from build123d import *

# Parameters (mm, degrees)
F0_R            = 4.05
F1_DEPTH        = 10
F2_R            = 5
F4_D            = 4.1000000042
F4_CSINK_D      = 7.7978
F4_CSINK_ANGLE  = 82
F5_W            = 1
F5_H            = 12
F6_DEPTH        = 0.4
F8_DEPTH        = 25
F10_D           = 3
F10_CBORE_D     = 6.5
F10_CBORE_DEPTH = 3


with BuildPart() as f1:
    # F0 (on Top) → F1 (new body)
    with BuildSketch(Plane.XY):
        Polygon((67.5994434953, -8.2149432153), (-62.4005565047, -8.2149432153), (-62.4005565047, -32.2149432153), (-28.9914757013, -32.2149432153), (-28.9914757013, -20.2149432153), (34.1903626919, -20.2149432153), (34.1903626919, -32.2149432153), (67.5994434953, -32.2149432153), align=None)
        with Locations((-47.4005565047, -20.2149432153)):
            Circle(F0_R, mode=Mode.SUBTRACT)
        with Locations((52.5994434953, -20.2149432153)):
            Circle(F0_R, mode=Mode.SUBTRACT)
    extrude(amount=F1_DEPTH)

    # F2
    f2_edges = [f1.edges().sort_by_distance(p)[0] for p in [
        (34.190363, -32.214943, 5),
        (-28.991476, -32.214943, 5),
    ]]
    fillet(f2_edges, radius=F2_R)

    # F4 (through all)
    with Locations(Plane.XZ.offset(20.2149432153)):
        with Locations((-18.9914757013, 5), (24.1903626919, 5)):
            CounterSinkHole(F4_D / 2, F4_CSINK_D / 2, counter_sink_angle=F4_CSINK_ANGLE)

    # F5 (on face) → F6 (join)
    with BuildSketch(Plane.XY.offset(10)):
        with Locations((2.5994434953, -14.2149432153)):
            Rectangle(F5_W, F5_H)
    extrude(amount=F6_DEPTH)

    # F7 (on face) → F8 (cut)
    with BuildSketch(Plane.XY.offset(10)):
        with BuildLine():
            ThreePointArc((56.6417200816, -19.9649432153), (56.6475121814, -20.0898835784), (56.6494434953, -20.2149432153))
            ThreePointArc((56.6494434953, -20.2149432153), (56.6475121814, -20.3400028521), (56.6417200816, -20.4649432153))
            Line((56.6417200816, -20.4649432153), (67.5994434953, -20.4649432153))
            Line((67.5994434953, -20.4649432153), (67.5994434953, -19.9649432153))
            Line((67.5994434953, -19.9649432153), (56.6417200816, -19.9649432153))
        make_face()
        with BuildLine():
            Line((-51.442833091, -19.9649432153), (-62.4005565047, -19.9649432153))
            Line((-62.4005565047, -19.9649432153), (-62.4005565047, -20.4649432153))
            Line((-62.4005565047, -20.4649432153), (-51.442833091, -20.4649432153))
            ThreePointArc((-51.442833091, -20.4649432153), (-51.4505565047, -20.2149432153), (-51.442833091, -19.9649432153))
        make_face()
        with BuildLine():
            Line((-51.442833091, -20.4649432153), (-51.442833091, -19.9649432153))
            ThreePointArc((-51.442833091, -19.9649432153), (-51.4505565047, -20.2149432153), (-51.442833091, -20.4649432153))
        make_face()
        with BuildLine():
            ThreePointArc((56.6417200816, -20.4649432153), (56.6475121814, -20.3400028521), (56.6494434953, -20.2149432153))
            ThreePointArc((56.6494434953, -20.2149432153), (56.6475121814, -20.0898835784), (56.6417200816, -19.9649432153))
            Line((56.6417200816, -19.9649432153), (56.6417200816, -20.4649432153))
        make_face()
    extrude(amount=-F8_DEPTH, mode=Mode.SUBTRACT)

    # F10 (through all)
    with Locations(Plane.XZ.offset(32.2149432153)):
        with Locations((61.5994434953, 5), (-56.4005565047, 5)):
            CounterBoreHole(F10_D / 2, F10_CBORE_D / 2, F10_CBORE_DEPTH)


solid = f1.part
Geometry: final body of the model. Coordinates: model frame, mm. A direction names the side the tool comes from. Coordinates: 2 decimals unless noted, no trailing zeros. Order: outer loops, then holes, each group sorted by start corner. A loop starts at its lowest first (then second) coordinate and runs counter-clockwise, first axis right, second up.
1) Section B-B (x = -45). Return loops of the section in (y, z), then the cut area to 3 significant figures.
Result sheet:
outline: (-32.21, 0) - (-23.48, 0) - (-23.48, 10) - (-32.21, 10) - close; (-16.95, 0) - (-8.21, 0) - (-8.21, 10) - (-16.95, 10) - close
area: 175 mm2
2) Ray query, probe 1 along Z at (x, y) = (61.5, -11); probe 2 along Y at (x, z) = (60, 2.5); probe 3 along X at (y, z) = (-22, 4). Return the intervals inside material, ascending.
Result sheet:
probe 1: z = 0 to 3.5, 6.5 to 10
probe 2: y = -29.21 to -20.46, -19.96 to -8.21
probe 3: x = -62.4 to -57.52, -55.28 to -51.04, -43.77 to -28.99, 34.19 to 48.96, 56.23 to 60.48, 62.72 to 67.6
3) First-contact query: P1, Ø5, axis at x = 61.6, z = 5, coming from the -Y side; P2, Ø6.5, axis at x = 52.6, y = -20.21, coming from the -Z side (1 decimal); P3, Ø2, axis at x = -39.5, y = -13.5, coming from the +Z side; P4, Ø1, axis at x = -17.5, z = 9, coming from the -Y side. Flat tips, straight axial feed; report the tip coordinate or a pass-through.
Result sheet:
P1: stops at y = -29.21
P2: passes through
P3: stops at z = 10
P4: stops at y = -20.21
4) Section A-A (y = -23). Return loops of the section in (x, z), then the cut area to 3 significant figures.
Result sheet:
outline: (-62.4, 0) - (-50.34, 0) - (-50.34, 10) - (-62.4, 10) - close; (-44.46, 0) - (-28.99, 0) - (-28.99, 10) - (-44.46, 10) - close; (34.19, 0) - (49.66, 0) - (49.66, 10) - (34.19, 10) - close; (55.54, 0) - (67.6, 0) - (67.6, 10) - (55.54, 10) - close; hole circle Ø3 at (-56.4, 5); hole circle Ø3 at (61.6, 5)
area: 536 mm2
5) Set-up query: faces 1 (the cylindrical face through (-59.647, -30.736, 5.143)), 2 (the flat face through (-31, -17, 10)), 3 (the flat face through (-62.401, -14, 5)), 4 (the flat face through (-28.991, -24, 5)). Return all of +Z, -Z, +X, -X, +Y, -Y with unobstructed straight access to the full face (end or side cutting, diameter ignored); none if empty.
Result sheet:
face 1: -Y
face 2: +Z, -X, +Y, -Y
face 3: +Z, -Z, -X, +Y, -Y
face 4: +Z, -Z, -Y
6) Draft query along Y for faces 5 (the flat face through (53, -32.215, 5)), 6 (the cylindrical face through (60.17, -14.01, 5.45)), 7 (the flat face through (-58.2, -20.465, 5.1)). Return one class per face: released by +Y, released by -Y, zero draft, split by the parting line, or undercut.
Result sheet:
face 5: released by -Y
face 6: zero draft
face 7: undercut
7) Section C-C (z = 5). Give the number of separate pieces and of enclosed holes in the cut face, then the cut area to 3 significant figures.
Result sheet:
separate pieces: 7
enclosed holes: 0
area: 1,970 mm2
8) Section D-D (x = 14.5). Return loops of the section in (y, z).
Result sheet:
outline: (-20.21, 0) - (-8.21, 0) - (-8.21, 10) - (-20.21, 10) - close
